Part model, mm, in its own coordinate system. A direction names the side the tool comes from. Give positions to 0.01 mm unless a question says otherwise; leave off trailing zeros. Loops run counter-clockwise (first coordinate to the right, second up) from the corner with the lowest first, then second, coordinate; pieces in that order, holes last. Notation, with made-up numbers: M -38,79.5 L 9,79.5 A18 cw 9,95.5 Z; hole C 8,77.25 d10. An arc over 180 degrees is marked long. Answer in a Markdown table with one row per item.
from build123d import *


with BuildPart() as part:
    # Sketch1 → Revolve1 (revolve)
    with BuildSketch(Plane.XY, mode=Mode.PRIVATE) as revolve1_sk:
        with BuildLine():
            Line((0, -4.03225), (0, 0))
            Line((0, 0), (34.925, 0))
            ThreePointArc((34.925, 0), (34.767418278, -0.418684593), (34.372884132, -0.629567487))
            Line((34.372884132, -0.629567487), (31.437637782, -1.016))
            Line((31.437637782, -1.016), (13.994321545, -1.016))
            Line((13.994321545, -1.016), (12.065, -1.27))
            Line((12.065, -1.27), (3.8608, -1.27))
            ThreePointArc((3.8608, -1.27), (1.558925, -2.037291667), (0.1778, -4.03225))
            Line((0.1778, -4.03225), (0, -4.03225))
        make_face()
    revolve(revolve1_sk.sketch.rotate(Axis((0, 0, 0), (1, 0, 0)), 270), axis=Axis((0, 0, 0), (1, 0, 0)))


solid = part.part
(1) Which spindle directions (+Z, -Z, +X, -X, +Y, -Y) get a long thin tool onto all of the face, cutting with end or side? Do faces 1 (the face through (22.59, 0.99, -0.22)), 2 (the face through (0, 0, 0)). Say none if no direction does.
Recorded:
| item | result |
|---|---|
| face 1 | +X |
| face 2 | +Z, -Z, -X, +Y, -Y |
(2) Pin check, flat tips, straight feed: pin 1 Ø4 at (x, y) = (9, -2) entering from +Z; pin 2 Ø3 at (x, y) = (29, 3) entering from +Z; pin 3 Ø4 at (x, z) = (19, 2.5) entering from +Y. Stop position of each tip, or through.
Recorded:
| item | result |
|---|---|
| pin 1 | stops at z = 1.27 |
| pin 2 | passes through |
| pin 3 | stops at y = 0.88 |
(3) Saw through at D-D (x = 3). Write the cut outline in (y, z), plus the area to 3 significant figures.
Recorded:
| item | result |
|---|---|
| outline | C 0,0 d2.74 |
| area | 5.88 mm^2 |
(4) Drill centre lines: line 1 along Y through (x, z) = (5.5, 0); line 2 along X through (y, z) = (-2.25, 0); line 3 along Z through (x, y) = (30.5, 0.5). Where is each one in solid material? Low to high.
Recorded:
| item | result |
|---|---|
| line 1 | y = -1.27 to 1.27 |
| line 2 | x = 0 to 1.3 |
| line 3 | z = -0.88 to 0.88 |
(5) Saw through at C-C (x = 21). Write the cut outline in (y, z), plus the area to 3 significant figures.
Recorded:
| item | result |
|---|---|
| outline | C 0,0 d2.03 |
| area | 3.24 mm^2 |
(6) Saw through at A-A (z = 0). Write the cut outline in (x, y) (3 decimals), plus the area to 3 significant figures.
Recorded:
| item | result |
|---|---|
| outline | M 0,-4.032 L 0.178,-4.032 A3.836 cw 3.861,-1.27 L 12.065,-1.27 L 13.994,-1.016 L 31.438,-1.016 L 34.373,-0.63 A0.635 ccw 34.373,0.63 L 31.438,1.016 L 13.994,1.016 L 12.065,1.27 L 3.861,1.27 A3.836 cw 0.178,4.032 L 0,4.032 Z |
| area | 82.2 mm^2 |
